Input: part model. Units: mm. Frame: model coordinates. A direction names the side the tool comes from. Round coordinates to 2 decimals unless told otherwise and drop trailing zeros. Order: outer loops, then holes, each group sorted by start corner. A loop starts at its lowest first (then second) coordinate and runs counter-clockwise, first axis right, second up. Notation, with made-up numbers: (-4.75, 82) -> (10.25, 82) arc R18 cw to (10.25, 98) -> close; hole circle Ø9 at (38, 57). An arc over 180 degrees is marked (long way). Use a Markdown table: item, result.
from build123d import *

# Parameters (mm, degrees)
SKETCH1_W                          = 38.1
SKETCH1_H                          = 63.5
BOSS_EXTRUDE1_DEPTH                = 3.175
SKETCH3_R                          = 3.302
SKETCH3_R_2                        = 1.016
HOLES_FOR_SERVO_MOUNT_DEPTH        = 4.175
SKETCH2_R                          = 1.7145
HOLES_FOR_TILT_SERVO_BRACKET_DEPTH = 4.175
SKETCH4_R                          = 1.7145
HOLES_FOR_PILLOW_BRACKET_DEPTH     = 4.175
SKETCH5_W                          = 8.89
SKETCH5_H                          = 17.78
CUT_EXTRUDE1_DEPTH                 = 4.175
SKETCH10_R                         = 1.7145
BOSS_EXTRUDE3_DEPTH                = 3.175


with BuildPart() as part:
    # Sketch1 → Boss-Extrude1 (new body)
    with BuildSketch(Plane(origin=(0, 0, 0), x_dir=(1, 0, 0), z_dir=(0, 1, 0))):
        Rectangle(SKETCH1_W, SKETCH1_H)
    extrude(amount=BOSS_EXTRUDE1_DEPTH)

    # Sketch3 → holes for servo mount (cut, through all)
    with BuildSketch(Plane(origin=(0, 3.175, 0), x_dir=(1, 0, 0), z_dir=(0, 1, 0))):
        with Locations((0.040685132, -9.433577206)):
            Circle(SKETCH3_R)
        with Locations((7.224890029, -16.617782103)):
            Circle(SKETCH3_R_2)
        with Locations((-7.143519765, -2.249372309)):
            Circle(SKETCH3_R_2)
        with Locations((-7.143519765, -16.617782103)):
            Circle(SKETCH3_R_2)
        with Locations((7.224890029, -2.249372309)):
            Circle(SKETCH3_R_2)
    extrude(amount=-HOLES_FOR_SERVO_MOUNT_DEPTH, mode=Mode.SUBTRACT)

    # Sketch2 → holes for tilt servo bracket (cut, through all)
    with BuildSketch(Plane(origin=(0, 3.175, 0), x_dir=(1, 0, 0), z_dir=(0, 1, 0))):
        with Locations((-6.071821378, 25.4)):
            Circle(SKETCH2_R)
        with Locations((6.628178622, 25.4)):
            Circle(SKETCH2_R)
        with Locations((6.628178622, -25.654)):
            Circle(SKETCH2_R)
        with Locations((-6.071821378, -25.654)):
            Circle(SKETCH2_R)
    extrude(amount=-HOLES_FOR_TILT_SERVO_BRACKET_DEPTH, mode=Mode.SUBTRACT)

    # Sketch4 → holes for pillow bracket (cut, through all)
    with BuildSketch(Plane(origin=(0, 3.175, 0), x_dir=(1, 0, 0), z_dir=(0, 1, 0))):
        with Locations((9.525, 9.652)):
            Circle(SKETCH4_R)
        with Locations((-9.525, 9.652)):
            Circle(SKETCH4_R)
    extrude(amount=-HOLES_FOR_PILLOW_BRACKET_DEPTH, mode=Mode.SUBTRACT)

    # Sketch5 → Cut-Extrude1 (cut, through all)
    with BuildSketch(Plane(origin=(0, 3.175, 0), x_dir=(1, 0, 0), z_dir=(0, 1, 0))):
        with Locations((-14.605, 22.86)):
            Rectangle(SKETCH5_W, SKETCH5_H)
    cut_extrude1 = extrude(amount=-CUT_EXTRUDE1_DEPTH, mode=Mode.SUBTRACT)

    # Mirror1: Cut-Extrude1 across plane
    add(cut_extrude1.mirror(Plane(origin=(0, 0, 0), x_dir=(0, 0, 1), z_dir=(1, 0, 0))), mode=Mode.SUBTRACT)

    # Sketch10 → Boss-Extrude3 (add)
    with BuildSketch(Plane(origin=(0, 3.175, 0), x_dir=(1, 0, 0), z_dir=(0, 1, 0))):
        Polygon((0, -31.75), (-10.16, -31.75), (-10.16, -50.073577206), (10.16, -50.073577206), (10.16, -31.75), align=None)
        with Locations((-6.071821378, -44.231577206)):
            Circle(SKETCH10_R, mode=Mode.SUBTRACT)
        with Locations((6.628178622, -44.231577206)):
            Circle(SKETCH10_R, mode=Mode.SUBTRACT)
    extrude(amount=-BOSS_EXTRUDE3_DEPTH)


solid = part.part
1) Cut plane A-A on z = -25.4. Return loops of the section in (x, y) (3 decimals).
Answer key:
| item | result |
|---|---|
| outline | (-10.16, 0) -> (-7.786, 0) -> (-7.786, 3.175) -> (-10.16, 3.175) -> close; (-4.357, 0) -> (4.914, 0) -> (4.914, 3.175) -> (-4.357, 3.175) -> close; (8.343, 0) -> (10.16, 0) -> (10.16, 3.175) -> (8.343, 3.175) -> close |
2) Contact query for flat-ended pins moving along their axis: P1, Ø4, axis at x = -6.07, z = 25.65, coming from the -Y side; P2, Ø1, axis at x = -15.5, y = 1, coming from the -Z side; P3, Ø1.6, axis at y = 2, z = -25.5, coming from the +X side; P4, Ø1, axis at x = -13.5, y = 2, coming from the +Z side. Output: stop coordinate, or through.
Answer key:
| item | result |
|---|---|
| P1 | stops at y = 0 |
| P2 | stops at z = -13.97 |
| P3 | stops at x = 10.16 |
| P4 | stops at z = 31.75 |
3) Set-up query: faces 1 (the face through (15, 2, 31.75)), 2 (the face through (-10.16, 2, -23)), 3 (the face through (10.16, 2, -23)), 4 (the face through (-15, 2, 31.75)). Return all of +Z, -Z, +X, -X, +Y, -Y with unobstructed straight access to the full face (end or side cutting, diameter ignored); none if empty.
Answer key:
| item | result |
|---|---|
| face 1 | +Z, +X, +Y, -Y |
| face 2 | -Z, -X, +Y, -Y |
| face 3 | -Z, +X, +Y, -Y |
| face 4 | +Z, -X, +Y, -Y |
4) Cut plane B-B on y = 1.4. State how many separate pieces and enclosed holes the cut face has, and give its area (3 significant figures).
Answer key:
| item | result |
|---|---|
| separate pieces | 1 |
| enclosed holes | 13 |
| area | 2,350 mm^2 |
5) Draft query along X for faces 5 (the face through (15, 2, -13.97)), 6 (the face through (10.316, 1.61, -8.131)), 7 (the face through (10.16, 2, 41)). Return one class per face: released by +X, released by -X, zero draft, split by the parting line, or undercut.
Answer key:
| item | result |
|---|---|
| face 5 | zero draft |
| face 6 | undercut |
| face 7 | released by +X |
6) Ray query, probe 1 along Z at (x, y) = (-6, 2.55); probe 2 along X at (y, z) = (0.9, -25.4); probe 3 along Z at (x, y) = (0, 2.2). Return the intervals inside material, ascending.
Answer key:
| item | result |
|---|---|
| probe 1 | z = -31.75 to -27.11, -23.69 to 23.94, 27.37 to 42.52, 45.94 to 50.07 |
| probe 2 | x = -10.16 to -7.79, -4.36 to 4.91, 8.34 to 10.16 |
| probe 3 | z = -31.75 to 6.13, 12.74 to 50.07 |
